```python
from build123d import *

# Parameters (mm, degrees)
BOSS_EXTRUDE1_DEPTH         = 25.4
C_0_242_DIAMETER_HOLE1_D    = 6.1468
F_1_4_0_25_DIAMETER_HOLE1_D = 6.35


with BuildPart() as part:
    # Sketch1 → Boss-Extrude1 (new body)
    with BuildSketch(Plane(origin=(0, 0, 0), x_dir=(1, 0, 0), z_dir=(0, 1, 0))):
        Polygon((0, 0), (0, 50.8), (50.8, 0), align=None)
        Polygon((3.175, 3.175), (3.175, 41.275), (41.275, 3.175), align=None, mode=Mode.SUBTRACT)
    extrude(amount=BOSS_EXTRUDE1_DEPTH)

    # C (0.242) Diameter Hole1 (through all)
    with Locations(Plane.ZY):
        with Locations((-12.7, 12.7), (-38.1, 12.7)):
            Hole(C_0_242_DIAMETER_HOLE1_D / 2)

    # 1/4 (0.25) Diameter Hole1 (through all)
    with Locations(Plane.XY):
        with Locations((38.1, 12.7), (12.7, 12.7)):
            Hole(F_1_4_0_25_DIAMETER_HOLE1_D / 2)


solid = part.part
```
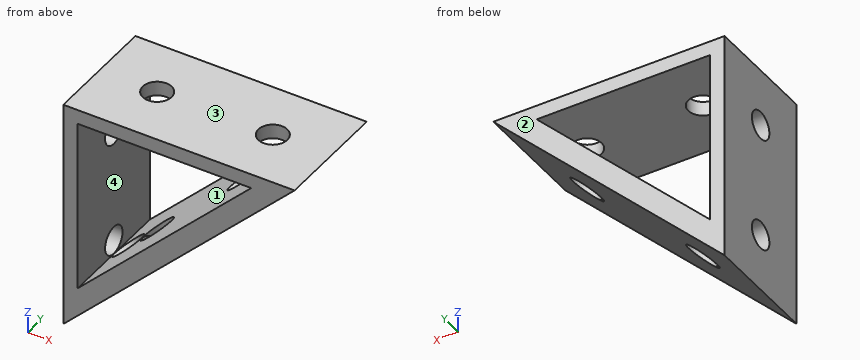
Can you work these out from the model? Positions are in its coordinate system, mm. Face numbers are marked on the shaded views. Round coordinates to 2 decimals unless told otherwise and drop trailing zeros. Loops run counter-clockwise (first coordinate to the right, second up) from the corner with the lowest first, then second, coordinate; pieces in that order, holes last. Notation, with made-up numbers: (-24.5, -20.75) -> (16.5, -20.75) arc R11 ccw to (16.5, -3.75) -> close; hole circle Ø5 at (77, -27.75). An arc over 180 degrees is marked (long way). Answer in a Markdown table with one row per item.
Item 1: Will these pins go through, and if not, where does the flat tip stop? P1, Ø10, axis at y = 9.5, z = -33, coming from the +X side; P2, Ø6, axis at x = 31.5, y = 22.5, coming from the +Z side; P3, Ø12.5, axis at x = 17, y = 17.5, coming from the -Z side; P4, Ø5.5, axis at y = 12.7, z = -12.7, coming from the +X side.
Answer block:
| item | result |
|---|---|
| P1 | x = 22.8 |
| P2 | z = 0 |
| P3 | z = -40.05 |
| P4 | through |
Item 2: Suppose I cut it at C-C, the plane z = -38.1. List the corners of the cut face in (x, y) for me (3 decimals), plus the area to 3 significant figures.
Answer block:
| item | result |
|---|---|
| outline | (0, 0) -> (3.175, 0) -> (3.175, 9.627) -> (0, 9.627) -> close; (0, 15.773) -> (3.175, 15.773) -> (3.175, 25.4) -> (0, 25.4) -> close; (6.35, 0) -> (12.7, 0) -> (12.7, 9.525) arc R3.175 cw to (11.903, 9.627) -> (6.35, 9.627) -> close; (6.35, 15.773) -> (11.903, 15.773) arc R3.175 cw to (12.7, 15.875) -> (12.7, 25.4) -> (6.35, 25.4) -> close |
| area | 183 mm² |
Item 3: We'd pull the mould along Z, two halves only. Please class the marked faces 1, 2, 3 and 4: released by +Z, released by -Z, zero draft, split by the parting line, or undercut.
Answer block:
| item | result |
|---|---|
| face 1 | undercut |
| face 2 | zero draft |
| face 3 | released by +Z |
| face 4 | undercut |
Item 4: Suppose I cut it at D-D, the plane y = 4.25. List the corners of the cut face in (x, z) for me (3 decimals).
Answer block:
| item | result |
|---|---|
| outline | (0, -50.8) -> (50.8, 0) -> (0, 0) -> close; hole (3.175, -41.275) -> (41.275, -3.175) -> (3.175, -3.175) -> close |
Item 5: If I drill on probe 1 along Y at (x, z) = (38.1, -11.25) (3 decimals); probe 2 along Y at (x, z) = (1.75, -38.1); probe 3 along Z at (x, y) = (33.75, 12.7) (3 decimals), over which ranges is the centre line in solid material (lowest first)?
Answer block:
| item | result |
|---|---|
| probe 1 | 0 to 9.525, 15.875 to 25.4 |
| probe 2 | 0 to 9.63, 15.77 to 25.4 |
| probe 3 | -17.05 to -15.773, -3.175 to 0 |
Item 6: Suppose I cut it at A-A, the plane x = 38.1. List the corners of the cut face in (y, z) for me (3 decimals), plus the area to 3 significant figures.
Answer block:
| item | result |
|---|---|
| outline | (0, -12.7) -> (9.525, -12.7) -> (9.525, -6.35) -> (0, -6.35) -> close; (0, -3.175) -> (9.525, -3.175) -> (9.525, 0) -> (0, 0) -> close; (15.875, -12.7) -> (25.4, -12.7) -> (25.4, -6.35) -> (15.875, -6.35) -> close; (15.875, -3.175) -> (25.4, -3.175) -> (25.4, 0) -> (15.875, 0) -> close |
| area | 181 mm² |
Item 7: Suppose I cut it at B-B, the plane z = -6. List the corners of the cut face in (x, y) for me (3 decimals).
Answer block:
| item | result |
|---|---|
| outline | (0, 0) -> (3.175, 0) -> (3.175, 25.4) -> (0, 25.4) -> close; (38.45, 0) -> (44.8, 0) -> (44.8, 25.4) -> (38.45, 25.4) -> (38.45, 15.856) arc R3.175 cw to (38.45, 9.544) -> close |
